Model file for the job. Use its own axes, mm. Face numbers are marked on the shaded views. A direction names the side the tool comes from. Give positions to 0.01 mm unless a question says otherwise; leave off trailing zeros. Loops run counter-clockwise (first coordinate to the right, second up) from the corner with the lowest first, then second, coordinate; pieces in that order, holes last. Notation, with made-up numbers: (-8, -3.75) - (22, -3.75) arc R32 ccw to (22, 25.25) - close; hole circle Ø11 at (-30.75, -10). An arc over 180 degrees is marked (long way). Use a Markdown table: item, result.
Autodesk Inventor part; units mm, degrees
ref_plane "YZ Plane" through (0, 0, 0) normal (1, 0, 0) x (0, 1, 0)
ref_plane "XZ Plane" through (0, 0, 0) normal (0, 1, 0) x (-1, 0, 0)
ref_plane "XY Plane" through (0, 0, 0) normal (0, 0, 1) x (1, 0, 0)
sketch "Эскиз1" plane through (0, 0, 0) normal (1, 0, 0) x (0, 1, 0)
  point P0 (0, 0)
sketch "Эскиз2" plane through (0, 0, 0) normal (0, 1, 0) x (-1, 0, 0)
  line L0 (19, -4) -> (-19, -4)
  line L1 (-19, -4) -> (-19, 4)
  line L2 (-19, 4) -> (19, 4)
  line L3 (19, 4) -> (19, -4)
  line L4 (19, -4) -> (-19, 4) construction
  line L5 (-19, -4) -> (19, 4) construction
  line L6 (19, 0) -> (-19, 0) construction
  circle A0 centre (-15, 0) radius 2
  line L7 (0, -4) -> (0, 4) construction
  circle A1 centre (15, 0) radius 2
  point P0 (0, 0)
  dimension "d1" = 30
  dimension "d2" = 4
  dimension "d3" = 38
  dimension "d4" = 8
extrude "Выдавливание1" add sketch "Эскиз2" along normal blind 35 contours L0 L1 L2 L3 | A0 | A1
fillet "Сопряжение1" radius 3.5 4 edges at (19, 17.5, 4) (19, 17.5, -4) (-19, 17.5, 4) (-19, 17.5, -4)
sketch "Эскиз3" plane through (-15.5, 0, 4) normal (0, 0, 1) x (1, 0, 0)
  line L0 (29, 35) -> (29, 0) construction
  line L1 (0, 0) -> (0, 35) construction
  line L2 (0, 0) -> (31, 0) construction
  line L3 (31, 35) -> (31, 0) construction
  line L4 (0, 35) -> (31, 35) construction
  line L5 (32, 35) -> (32, 0) construction
  line L6 (34.5, 35) -> (31, 35) construction
  line L7 (31, 35) -> (31, 0) construction
  line L8 (31, 0) -> (34.5, 0) construction
  line L9 (34.5, 0) -> (34.5, 35) construction
  line L10 (-1, 35) -> (-1, 0) construction
  line L11 (0, 35) -> (-3.5, 35) construction
  line L12 (-3.5, 35) -> (-3.5, 0) construction
  line L13 (-3.5, 0) -> (0, 0) construction
  line L14 (0, 0) -> (0, 35) construction
  line L15 (0, 0) -> (0, 35) construction
  line L16 (-1, 35) -> (2, 35) construction
  line L17 (29, 35) -> (32, 35) construction
  line L18 (29, 0) -> (32, 0) construction
  line L19 (-1, 35) -> (2, 35) construction
  line L20 (-1, 0) -> (2, 0) construction
  line L21 (-1, 35) -> (2, 35) construction
  line L22 (-1, 0) -> (2, 0) construction
  line L23 (2, 35) -> (2, 0) construction
  line L24 (29, 35) -> (2, 0) construction
  line L25 (2, 35) -> (29, 0) construction
  line L26 (15.5, 17.5) -> (15.5, 35) construction
  line L27 (0, 35) -> (31, 35) construction
  circle A0 centre (15.5, 12) radius 10.5
  point P0 (15.5, 0)
  dimension "d8" = 21
  dimension "d9" = 12
extrude "Выдавливание2" cut sketch "Эскиз3" against normal blind 35
sketch "Эскиз4" plane through (-15.5, 0, 4) normal (0, 0, 1) x (1, 0, 0)
  circle A0 centre (15.5, 12) radius 10.5 construction
  circle A1 centre (15.5, 12) radius 10.5 construction
  line L0 (0, 0) -> (0, 35) construction
  line L1 (0, 0) -> (31, 0) construction
  line L2 (31, 35) -> (31, 0) construction
  line L3 (0, 35) -> (31, 35) construction
  line L4 (-1, 35) -> (-1, 0) construction
  line L5 (0, 35) -> (-3.5, 35) construction
  line L6 (-3.5, 35) -> (-3.5, 0) construction
  line L7 (-3.5, 0) -> (0, 0) construction
  line L8 (0, 0) -> (0, 35) construction
  line L9 (34.5, 35) -> (31, 35) construction
  line L10 (31, 35) -> (31, 0) construction
  line L11 (31, 0) -> (34.5, 0) construction
  line L12 (34.5, 0) -> (34.5, 35) construction
  arc A2 (-1, 2.5793) -> (34.5, 12) centre (15.5, 12) ccw construction
  line L13 (-3.5, 0) -> (-3.5, 35) construction
  line L14 (34.5, 0) -> (34.5, 35) construction
  arc A3 (-3.5, 12) -> (-1, 2.5793) centre (15.5, 12) ccw construction
  arc A4 (34.5, 12) -> (-3.5, 12) centre (15.5, 12) ccw
  line L15 (-3.5, 12) -> (-17.3538, 35.9689)
  line L16 (-17.3538, 35.9689) -> (7.0238, 39.959)
  line L17 (7.0238, 39.959) -> (47.0337, 39.6857)
  line L18 (47.0337, 39.6857) -> (34.5, 12)
  point P0 (15.5, 0)
extrude "Выдавливание3" cut sketch "Эскиз4" against normal blind 35
sketch "Эскиз5" plane through (0, 0, 0) normal (0, -1, 0) x (1, 0, 0)
  circle A0 centre (-15, 0) radius 2
  circle A1 centre (15, 0) radius 2
  point P0 (0, 0)
extrude "Выдавливание4" cut sketch "Эскиз5" against normal blind 12
properties part number "mid_mount_v2" material "Пластик АБС"
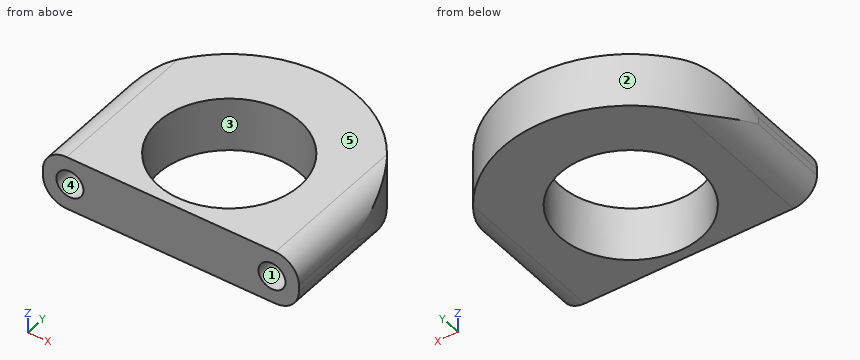
(1) Slice it at D-D, the plane x = 8. Write the cut outline in (y, z), plus the area to 3 significant figures.
Computed:
| item | result |
|---|---|
| outline | (0, -4) - (5.2, -4) - (5.2, 4) - (0, 4) - close; (18.8, -4) - (29.23, -4) - (29.23, 4) - (18.8, 4) - close |
| area | 125 mm² |
(2) Slice it at A-A, the plane x = 0. Write the cut outline in (y, z).
Computed:
| item | result |
|---|---|
| outline | (0, -4) - (1.5, -4) - (1.5, 4) - (0, 4) - close; (22.5, -4) - (31, -4) - (31, 4) - (22.5, 4) - close |
(3) Slice it at B-B, the plane z = 0. Write the cut outline in (x, y).
Computed:
| item | result |
|---|---|
| outline | (-19, 0) - (-17, 0) - (-17, 12) - (-13, 12) - (-13, 0) - (13, 0) - (13, 12) - (17, 12) - (17, 0) - (19, 0) - (19, 12) arc R19 ccw to (-19, 12) - close; hole circle Ø21 at (0, 12) |
(4) Mould opens along Y. For the marked faces 1, 2 and 3 say: pulls with the +Y half, pulls with the -Y half, needs draft (parallel to the pull), parting line crosses it, or undercut.
Computed:
| item | result |
|---|---|
| face 1 | needs draft |
| face 2 | pulls with the +Y half |
| face 3 | undercut |
(5) Slice it at C-C, the plane y = 19.5. Write the cut outline in (x, z), plus the area to 3 significant figures.
Computed:
| item | result |
|---|---|
| outline | (-17.46, -3.4) arc R3.5 ccw to (-15.5, -4) - (-7.35, -4) - (-7.35, 4) - (-15.5, 4) arc R3.5 ccw to (-17.46, 3.4) - close; (7.35, -4) - (15.5, -4) arc R3.5 ccw to (17.46, -3.4) - (17.46, 3.4) arc R3.5 ccw to (15.5, 4) - (7.35, 4) - close |
| area | 160 mm² |
(6) Pin check, flat tips, straight feed: P1, Ø2, axis at y = 5, z = 2, coming from the -X side; P2, Ø2.5, axis at x = -15, z = 0, coming from the +Y side; P3, Ø2, axis at x = -15.5, z = -0.5, coming from the -Y side. Stop position of each tip, or through.
Computed:
| item | result |
|---|---|
| P1 | x = -18.96 |
| P2 | y = 25.11 |
| P3 | y = 12 |
(7) 3-axis set-ups, long thin cutter, end or side, ignore diameter. For the marked faces 4 and 5: which of +Z, -Z, +X, -X, +Y, -Y reach the whole face in a straight line?
Computed:
| item | result |
|---|---|
| face 4 | -Y |
| face 5 | +Z, +X, -X, +Y, -Y |
(8) Drill centre lines: probe 1 along Z at (x, y) = (15, 8); probe 2 along X at (y, z) = (21, 0.75); probe 3 along X at (y, z) = (19.5, 3.25). Where is each one in solid material? Low to high. Write a range as [from, to].
Computed:
| item | result |
|---|---|
| probe 1 | [-4, -2], [2, 4] |
| probe 2 | [-16.73, -5.41], [5.41, 16.73] |
| probe 3 | [-17.46, -7.35], [7.35, 17.46] |
